Here's the drawing with two shaded views (mm, measured from the low corner). I have some questions. A direction names the side the tool comes from. Give positions to 0.01 mm unless a question says otherwise; leave off trailing zeros. Loops run counter-clockwise (first coordinate to the right, second up) from the corner with the lowest first, then second, coordinate; pieces in that order, holes last. Notation, with made-up numbers: (31, -33) -> (87, -33) arc R9 ccw to (87, -18) -> close; hole circle Ø6 at (50.25, 49.25). An arc over 180 degrees is marked (long way). Put each result on its own line as item: value.
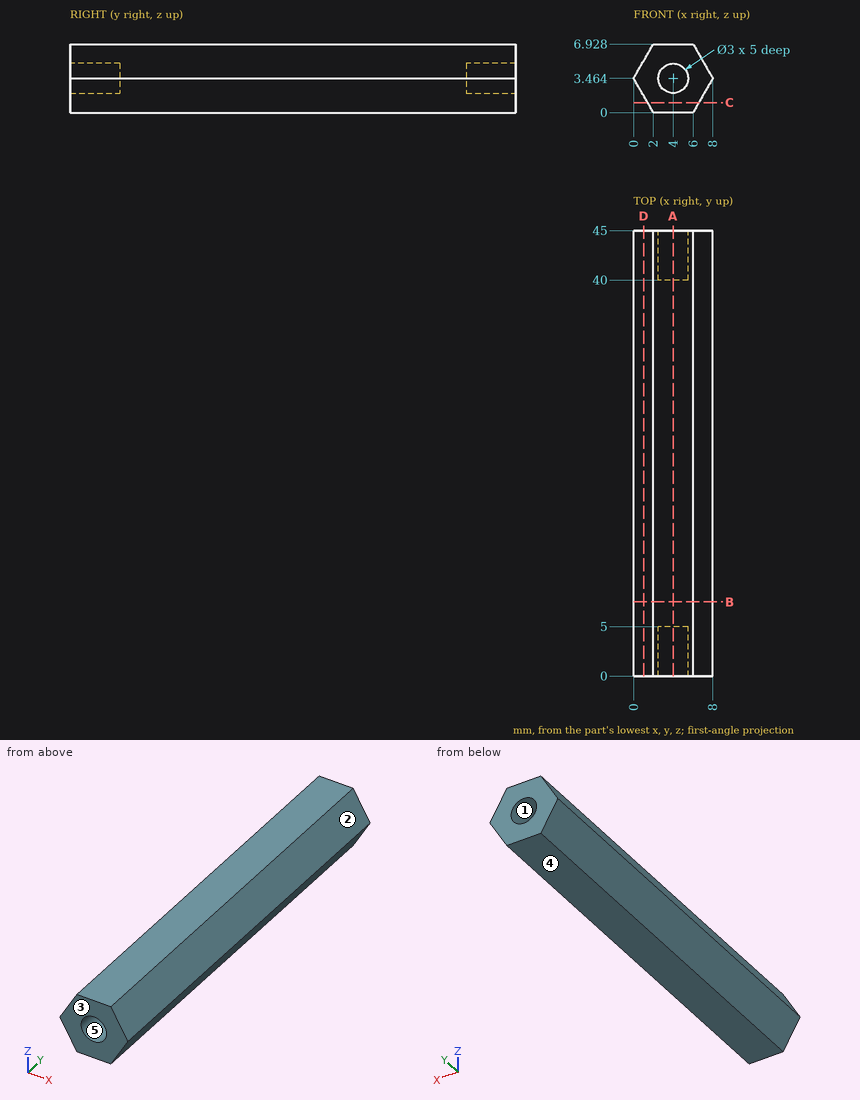
1. If we section it at A-A (x = 4): List the corners of the cut face in (y, z) for me.
Recorded:
outline: (0, 0) -> (45, 0) -> (45, 1.96) -> (40, 1.96) -> (40, 4.96) -> (45, 4.96) -> (45, 6.93) -> (0, 6.93) -> (0, 4.96) -> (5, 4.96) -> (5, 1.96) -> (0, 1.96) -> close
2. I'm going to push flat-ended pins straight in: pin 1 (4 mm diameter, centred on y = 23.5, z = 5, fed in from +X); pin 2 (4 mm diameter, centred on y = 31.5, z = 2.5, fed in from -X); pin 3 (2.5 mm diameter, centred on x = 4, z = 3.46, fed in from +Y). Where does each tip first touch, or does it pass through?
Recorded:
pin 1: stops at x = 8
pin 2: stops at x = 0
pin 3: stops at y = 40
3. If we section it at B-B (y = 7.5): List the corners of the cut face in (x, z) for me, then the cut area to 3 significant figures.
Recorded:
outline: (0, 3.46) -> (2, 0) -> (6, 0) -> (8, 3.46) -> (6, 6.93) -> (2, 6.93) -> close
area: 41.6 mm^2
4. I need wall thicknesses on line 1 (Y direction, x = 4.25, z = 4.75); line 2 (Z direction, x = 6.75, y = 40); line 3 (X direction, y = 20.5, z = 0.5). Which ranges of each line are inside material? Lowest first, please.
Recorded:
line 1: y = 5 to 40
line 2: z = 1.3 to 5.63
line 3: x = 1.71 to 6.29
5. Thinking about a two-plate mould opening in X: for the marked faces 1, 2 and 3, which applies, pulls with the +X half, pulls with the -X half, needs draft (parallel to the pull), parting line crosses it, or undercut?
Recorded:
face 1: undercut
face 2: pulls with the +X half
face 3: needs draft
6. If we section it at D-D (x = 1): List the corners of the cut face in (y, z) for me, then the cut area to 3 significant figures.
Recorded:
outline: (0, 1.73) -> (45, 1.73) -> (45, 5.2) -> (0, 5.2) -> close
area: 156 mm^2
7. If we section it at C-C (z = 1): List the corners of the cut face in (x, y) for me.
Recorded:
outline: (1.42, 0) -> (6.58, 0) -> (6.58, 45) -> (1.42, 45) -> close
8. For the marked faces 4 and 5, which set-ups out of +Z, -Z, +X, -X, +Y, -Y let a thin tool reach every point of the face, with its end or its side?
Recorded:
face 4: -Z, +X, -X, +Y, -Y
face 5: -Y
